```python
from build123d import *

# Parameters (mm, degrees)
SKETCH_1_W          = 80
SKETCH_1_H          = 40
EXTRUDE_1_DEPTH     = 50
CUT_EXTRUDE_1_DEPTH = 81
SKETCH_3_W          = 20
SKETCH_3_H          = 6
CUT_EXTRUDE_2_DEPTH = 81
SKETCH_4_W          = 5
SKETCH_4_H          = 8
CUT_EXTRUDE_3_DEPTH = 81


with BuildPart() as part:
    # 草图1 → 凸台-拉伸1 (new body)
    with BuildSketch(Plane(origin=(0, 0, 0), x_dir=(1, 0, 0), z_dir=(0, 1, 0))):
        Rectangle(SKETCH_1_W, SKETCH_1_H)
    extrude(amount=EXTRUDE_1_DEPTH)

    # 草图2 → 切除-拉伸1 (cut, symmetric)
    with BuildSketch(Plane.XY):
        Polygon((-20, 50), (20, 50), (2, 32), (2, 26), (-2, 26), (-2, 32), align=None)
    extrude(amount=CUT_EXTRUDE_1_DEPTH, both=True, mode=Mode.SUBTRACT)

    # 草图3 → 切除-拉伸2 (cut, symmetric)
    with BuildSketch(Plane.XY):
        with Locations((0, 3)):
            Rectangle(SKETCH_3_W, SKETCH_3_H)
    extrude(amount=CUT_EXTRUDE_2_DEPTH, both=True, mode=Mode.SUBTRACT)

    # 草图4 → 切除-拉伸3 (cut, symmetric)
    with BuildSketch(Plane.XY):
        with Locations((-37.5, 34)):
            Rectangle(SKETCH_4_W, SKETCH_4_H)
        with Locations((37.5, 34)):
            Rectangle(SKETCH_4_W, SKETCH_4_H)
    extrude(amount=CUT_EXTRUDE_3_DEPTH, both=True, mode=Mode.SUBTRACT)


solid = part.part
```
The listing builds one solid part. Answer for the finished solid, in the listing's coordinates (mm). A direction names the side the tool comes from. Round coordinates to 2 decimals unless told otherwise and drop trailing zeros. Write each loop counter-clockwise with the first axis right and the second up, starting at its lowest first coordinate (ties: lowest second). Pieces come first, ordered by that corner, then holes. Notation, with made-up numbers: (59, 15.25) -> (85, 15.25) arc R33 cw to (85, 52.25) -> close; hole circle Ø6 at (76.5, 47.25). An arc over 180 degrees is marked (long way). Answer as a JSON object with one key per item and string values. Group by question number.
Q1. Determine the mould class of faces 4 (the face through (-2, 29, 0)), 5 (the face through (-10, 3, 0)), 6 (the face through (40, 44, 0)), 7 (the face through (37, 30, 0)) for opening direction X: pulls with the +X half, pulls with the -X half, needs draft (parallel to the pull), parting line crosses it, or undercut.
Q2. Section C-C (y = 36) is taken. Write down the section's boundary in (x, z), plus the area to 3 significant figures.
Q3. Section B-B (z = -3) is taken. Write down the section's boundary in (x, y).
Q4. This flat-tipped pin is pushed along its axis until it touches: pin 1 Ø6 at (x, z) = (-3.5, -5) entering from -Y. Where does it stop, or does it pass through?
Q5. Straight lines are drawn through the part: line 1 along X through (y, z) = (4, 1.5); line 2 along X through (y, z) = (42.5, -11.5); line 3 along Y through (x, z) = (-14.5, -10.5). For each, find the intervals that lie inside material, in ascending order.
Q6. Which of the six approach directions +Z, -Z, +X, -X, +Y, -Y give full straight-line access (tool end or side, diameter ignored) to faces 1 (the face through (35, 34, 0)), 2 (the face through (-35, 34, 0)), 3 (the face through (0, 26, 0))?
Q7. Section D-D (x = 6) is taken. Write down the section's boundary in (y, z).
Q8. Section A-A (y = 3) is taken. Write down the section's boundary in (x, z).
Check values:
{
 "1": {"face 4": "undercut", "face 5": "undercut", "face 6": "pulls with the +X half", "face 7": "needs draft"},
 "2": {"outline": "(-35, -20) -> (-6, -20) -> (-6, 20) -> (-35, 20) -> close; (6, -20) -> (35, -20) -> (35, 20) -> (6, 20) -> close", "area": "2,320 mm^2"},
 "3": {"outline": "(-40, 0) -> (-10, 0) -> (-10, 6) -> (10, 6) -> (10, 0) -> (40, 0) -> (40, 30) -> (35, 30) -> (35, 38) -> (40, 38) -> (40, 50) -> (20, 50) -> (2, 32) -> (2, 26) -> (-2, 26) -> (-2, 32) -> (-20, 50) -> (-40, 50) -> (-40, 38) -> (-35, 38) -> (-35, 30) -> (-40, 30) -> close"},
 "4": {"pin 1": "y = 6"},
 "5": {"line 1": "-40 to -10, 10 to 40", "line 2": "-40 to -12.5, 12.5 to 40", "line 3": "0 to 44.5"},
 "6": {"face 1": "+Z, -Z, +X", "face 2": "+Z, -Z, -X", "face 3": "+Z, -Z, +Y"},
 "7": {"outline": "(6, -20) -> (36, -20) -> (36, 20) -> (6, 20) -> close"},
 "8": {"outline": "(-40, -20) -> (-10, -20) -> (-10, 20) -> (-40, 20) -> close; (10, -20) -> (40, -20) -> (40, 20) -> (10, 20) -> close"}
}
